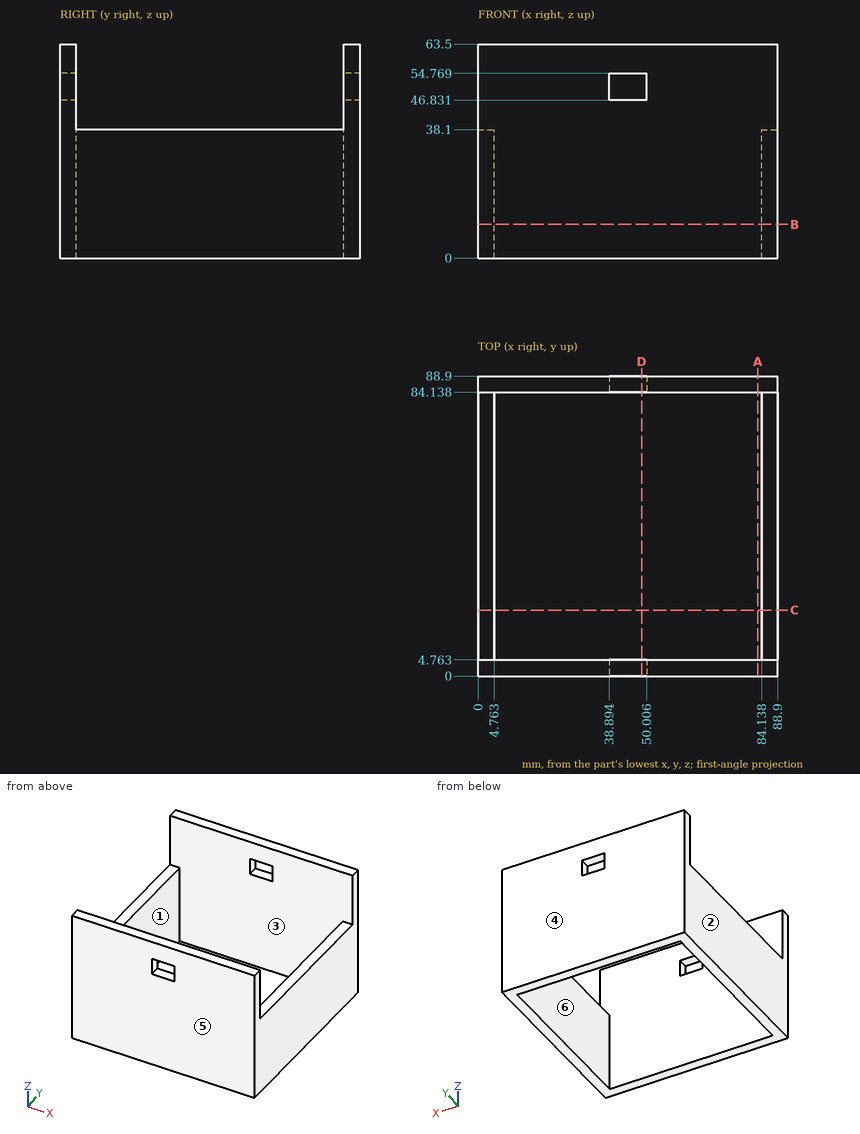
Here's the drawing with two shaded views (mm, measured from the low corner). I have some questions. A direction names the side the tool comes from. Give positions to 0.01 mm unless a question says otherwise; leave off trailing zeros. Order: outer loops, then holes, each group sorted by start corner. A loop starts at its lowest first (then second) coordinate and runs counter-clockwise, first axis right, second up. Notation, with made-up numbers: M -9.75,61.25 L 42.25,61.25 A35 ccw 42.25,94.25 Z; hole C 8.25,85 d6. An arc over 180 degrees is marked long. One line per item, written item: value.
1) I want a section at C-C, the plane y = 19.5. List the corners of the cut face in (x, z) for me, plus the area to 3 significant figures.
Answer sheet:
outline: M 0,0 L 4.76,0 L 4.76,38.1 L 0,38.1 Z; M 84.14,0 L 88.9,0 L 88.9,38.1 L 84.14,38.1 Z
area: 363 mm^2
2) For P1, Ø5, axis at x = 3.5, y = 32, coming from the +Z side, with a flat end and sliding along its axis, tell me the tip position at first contact or that it passes through.
Answer sheet:
P1: stops at z = 38.1
3) I want a section at D-D, the plane x = 48.5. List the corners of the cut face in (y, z) for me.
Answer sheet:
outline: M 0,0 L 4.76,0 L 4.76,46.83 L 0,46.83 Z; M 0,54.77 L 4.76,54.77 L 4.76,63.5 L 0,63.5 Z; M 84.14,0 L 88.9,0 L 88.9,46.83 L 84.14,46.83 Z; M 84.14,54.77 L 88.9,54.77 L 88.9,63.5 L 84.14,63.5 Z
4) We'd pull the mould along Y, two halves only. Please class the marked faces 1, 2, 3 and 4: released by +Y, released by -Y, zero draft, split by the parting line, or undercut.
Answer sheet:
face 1: undercut
face 2: zero draft
face 3: undercut
face 4: released by +Y
5) On a 3-axis mill with a long thin cutter (end or side, diameter ignored), from which of +Z, -Z, +X, -X, +Y, -Y can I reach the whole of each face in a straight line? I mean the marked faces 5 and 6. Say none if no direction works.
Answer sheet:
face 5: +Z, -Z, +X, -X, -Y
face 6: +Z, -Z
6) Please list where this line runs through material, in increasing order: line 1 along X through (y, z) = (52, 21.5).
Answer sheet:
line 1: x = 0 to 4.76, 84.14 to 88.9
7) I want a section at A-A, the plane x = 83. List the corners of the cut face in (y, z) for me.
Answer sheet:
outline: M 0,0 L 4.76,0 L 4.76,63.5 L 0,63.5 Z; M 84.14,0 L 88.9,0 L 88.9,63.5 L 84.14,63.5 Z
8) I want a section at B-B, the plane z = 10. List the corners of the cut face in (x, y) for me, plus the area to 3 significant figures.
Answer sheet:
outline: M 0,0 L 88.9,0 L 88.9,88.9 L 0,88.9 Z; hole M 4.76,4.76 L 84.14,4.76 L 84.14,84.14 L 4.76,84.14 Z
area: 1,600 mm^2
